Model file for the job. Use its own axes, mm. Face numbers are marked on the shaded views. A direction names the side the tool comes from. Round coordinates to 2 decimals unless told otherwise and drop trailing zeros. Write each loop counter-clockwise with the first axis right and the second up, starting at its lowest first coordinate (ties: lowest second). Pieces come first, ordered by that corner, then holes. Notation, with made-up numbers: (9, 66.25) - (16, 66.25) arc R16 ccw to (16, 72.25) - close; hole circle Ø11 at (-34.5, 74.25). An arc over 180 degrees is marked (long way). One line per item, written item: value.
from build123d import *
from OCP.BRepFilletAPI import BRepFilletAPI_MakeChamfer

# Parameters (mm, degrees)
SKETCH_184_R           = 15
EXTRUDE_842_DEPTH      = 3.5
CUT_EXTRUDE_1179_DEPTH = 2.7
CHAMFER_1_SIZE         = 0.5
CHAMFER_1_SIZE2        = 0.866025404


with BuildPart() as part:
    # Sketch 184 → Extrude 842 (new body)
    with BuildSketch(Plane.XY):
        Circle(SKETCH_184_R)
        with BuildLine():
            Line((4.5, 2.75), (4.5, -2.75))
            ThreePointArc((4.5, -2.75), (0, -7.25), (-4.5, -2.75))
            Line((-4.5, -2.75), (-4.5, 2.75))
            ThreePointArc((-4.5, 2.75), (0, 7.25), (4.5, 2.75))
        make_face(mode=Mode.SUBTRACT)
    extrude(amount=EXTRUDE_842_DEPTH)

    # Эскиз1 → Cut-Extrude 1179 (cut)
    with BuildSketch(Plane.XY.offset(3.5)):
        with BuildLine():
            Line((6.6, 2.45), (6.6, -2.45))
            ThreePointArc((6.6, -2.45), (0, -9.05), (-6.6, -2.45))
            Line((-6.6, -2.45), (-6.6, 2.45))
            ThreePointArc((-6.6, 2.45), (0, 9.05), (6.6, 2.45))
        make_face()
    extrude(amount=-CUT_EXTRUDE_1179_DEPTH, mode=Mode.SUBTRACT)

    # Фаска1: one chamfer whose edges measure the first distance from different faces: ONE call of the kernel's chamfer builder (chamfer() names one face for all edges)
    chamfer_1_edges_1 = [part.edges().sort_by_distance(p)[0] for p in [
        (-15, 0, 0),
    ]]
    chamfer_1_side_1 = [part.faces().sort_by_distance(p)[0] for p in [
        (-14.575735931, 0, 0),
    ]]
    chamfer_1_edges_2 = [part.edges().sort_by_distance(p)[0] for p in [
        (0, 7.25, 0),
    ]]
    chamfer_1_side_2 = [part.faces().sort_by_distance(p)[0] for p in [
        (0, 7.25, 0.4),
    ]]
    chamfer_1_edges_3 = [part.edges().sort_by_distance(p)[0] for p in [
        (-4.5, 0, 0),
    ]]
    chamfer_1_side_3 = [part.faces().sort_by_distance(p)[0] for p in [
        (-4.5, 0, 0.4),
    ]]
    chamfer_1_edges_4 = [part.edges().sort_by_distance(p)[0] for p in [
        (0, -7.25, 0),
    ]]
    chamfer_1_side_4 = [part.faces().sort_by_distance(p)[0] for p in [
        (0, -7.25, 0.4),
    ]]
    chamfer_1_edges_5 = [part.edges().sort_by_distance(p)[0] for p in [
        (4.5, 0, 0),
    ]]
    chamfer_1_side_5 = [part.faces().sort_by_distance(p)[0] for p in [
        (4.5, 0, 0.4),
    ]]
    chamfer_1 = BRepFilletAPI_MakeChamfer(part.part.solid().wrapped)
    for e in chamfer_1_edges_1:
        chamfer_1.Add(CHAMFER_1_SIZE, CHAMFER_1_SIZE2, e.wrapped, chamfer_1_side_1[0].wrapped)  # the first distance lies on this face
    for e in chamfer_1_edges_2:
        chamfer_1.Add(CHAMFER_1_SIZE, CHAMFER_1_SIZE2, e.wrapped, chamfer_1_side_2[0].wrapped)  # the first distance lies on this face
    for e in chamfer_1_edges_3:
        chamfer_1.Add(CHAMFER_1_SIZE, CHAMFER_1_SIZE2, e.wrapped, chamfer_1_side_3[0].wrapped)  # the first distance lies on this face
    for e in chamfer_1_edges_4:
        chamfer_1.Add(CHAMFER_1_SIZE, CHAMFER_1_SIZE2, e.wrapped, chamfer_1_side_4[0].wrapped)  # the first distance lies on this face
    for e in chamfer_1_edges_5:
        chamfer_1.Add(CHAMFER_1_SIZE, CHAMFER_1_SIZE2, e.wrapped, chamfer_1_side_5[0].wrapped)  # the first distance lies on this face
    add(Compound.cast(chamfer_1.Shape()), mode=Mode.REPLACE)


solid = part.part
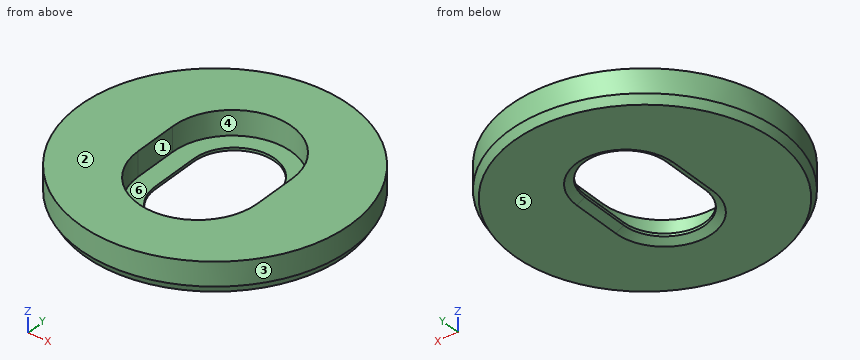
1. Mould opens along X. For the marked faces 1, 2, 3 and 4 say: released by +X, released by -X, zero draft, split by the parting line, or undercut.
Report:
face 1: undercut
face 2: zero draft
face 3: split by the parting line
face 4: undercut
2. Drop flat-ended pins along their axis: pin 1 (4 mm diameter, centred on x = 3, y = 4, fed in from +Z); pin 2 (1.5 mm diameter, centred on y = 4.5, z = 2, fed in from -X); pin 3 (2 mm diameter, centred on y = 6, z = 2, fed in from +X); pin 4 (8 mm diameter, centred on x = 2, y = -7.5, fed in from +Z). Give the stop position or say it passes through.
Report:
pin 1: z = 0.8
pin 2: x = -14.52
pin 3: x = 14.14
pin 4: z = 3.5
3. Band-saw the part on B-B on x = 0. Write the cut outline in (y, z), plus the area to 3 significant figures.
Report:
outline: (-15, 0.87) - (-14.5, 0) - (-8.12, 0) - (-7.25, 0.5) - (-7.25, 0.8) - (-9.05, 0.8) - (-9.05, 3.5) - (-15, 3.5) - close; (7.25, 0.5) - (8.12, 0) - (14.5, 0) - (15, 0.87) - (15, 3.5) - (9.05, 3.5) - (9.05, 0.8) - (7.25, 0.8) - close
area: 43.7 mm²
4. Wall check: probe 1 along Z at (x, y) = (-5.5, -6); probe 2 along Y at (x, z) = (-1.5, 2.7); probe 3 along Y at (x, z) = (-1, 0.55). Give the ranges that are in metal, low to high. Write a range as [from, to].
Report:
probe 1: [0, 0.8]
probe 2: [-14.92, -8.88], [8.88, 14.92]
probe 3: [-14.78, -7.14], [7.14, 14.78]
5. Band-saw the part on A-A on y = 0. Write the cut outline in (x, z), plus the area to 3 significant figures.
Report:
outline: (-15, 0.87) - (-14.5, 0) - (-5.37, 0) - (-4.5, 0.5) - (-4.5, 0.8) - (-6.6, 0.8) - (-6.6, 3.5) - (-15, 3.5) - close; (4.5, 0.5) - (5.37, 0) - (14.5, 0) - (15, 0.87) - (15, 3.5) - (6.6, 3.5) - (6.6, 0.8) - (4.5, 0.8) - close
area: 61.3 mm²
6. Tool access for the marked faces 5 and 6: list every direction of +Z, -Z, +X, -X, +Y, -Y with a clear straight run to the whole face (end or side of a thin tool).
Report:
face 5: -Z, +X, -X, +Y, -Y
face 6: +Z
7. Band-saw the part on C-C on z = 2.5. Write the cut outline in (x, y), plus the area to 3 significant figures.
Report:
outline: circle Ø30 at (0, 0); hole (-6.6, -2.45) arc R6.6 ccw to (6.6, -2.45) - (6.6, 2.45) arc R6.6 ccw to (-6.6, 2.45) - close
area: 505 mm²
